```python
from build123d import *

# Parameters (mm, degrees)
SKETCH1_W           = 240
SKETCH1_H           = 45
SKETCH1_R           = 1.5
SKETCH1_W_2         = 5
SKETCH1_H_2         = 10
BOSS_EXTRUDE1_DEPTH = 5
CUT_EXTRUDE1_DEPTH  = 5
FILLET1_R           = 2
CONG_1_R            = 5


with BuildPart() as part:
    # Sketch1 → Boss-Extrude1 (new body)
    with BuildSketch(Plane.XY):
        with Locations((34.186746988, 0)):
            Rectangle(SKETCH1_W, SKETCH1_H)
        with Locations((-78.313253012, 0)):
            Circle(SKETCH1_R, mode=Mode.SUBTRACT)
        with Locations(Location((146.686746988, 0, 0), (0, 0, 180))):
            Circle(SKETCH1_R, mode=Mode.SUBTRACT)
        with Locations((-78.313253012, -15)):
            Rectangle(SKETCH1_W_2, SKETCH1_H_2, mode=Mode.SUBTRACT)
        with Locations((-78.313253012, 15)):
            Rectangle(SKETCH1_W_2, SKETCH1_H_2, mode=Mode.SUBTRACT)
        with Locations((146.686746988, -15)):
            Rectangle(SKETCH1_W_2, SKETCH1_H_2, mode=Mode.SUBTRACT)
        with Locations((146.686746988, 15)):
            Rectangle(SKETCH1_W_2, SKETCH1_H_2, mode=Mode.SUBTRACT)
    extrude(amount=BOSS_EXTRUDE1_DEPTH)

    # Sketch2 → Cut-Extrude1 (cut)
    with BuildSketch(Plane.XY.offset(5)):
        with BuildLine():
            Line((-68.813253012, 22.5), (-62.813253012, 22.5))
            Line((-62.813253012, 22.5), (-64.063253012, 10))
            ThreePointArc((-64.063253012, 10), (-65.813253012, 8.25), (-67.563253012, 10))
            Line((-67.563253012, 10), (-68.813253012, 22.5))
        make_face()
        with BuildLine():
            Line((-43.813253012, 22.5), (-37.813253012, 22.5))
            Line((-37.813253012, 22.5), (-39.063253012, 10))
            ThreePointArc((-39.063253012, 10), (-40.813253012, 8.25), (-42.563253012, 10))
            Line((-42.563253012, 10), (-43.813253012, 22.5))
        make_face()
        with BuildLine():
            Line((-18.813253012, 22.5), (-12.813253012, 22.5))
            Line((-12.813253012, 22.5), (-14.063253012, 10))
            ThreePointArc((-14.063253012, 10), (-15.813253012, 8.25), (-17.563253012, 10))
            Line((-17.563253012, 10), (-18.813253012, 22.5))
        make_face()
        with BuildLine():
            Line((6.186746988, 22.5), (12.186746988, 22.5))
            Line((12.186746988, 22.5), (10.936746988, 10))
            ThreePointArc((10.936746988, 10), (9.186746988, 8.25), (7.436746988, 10))
            Line((7.436746988, 10), (6.186746988, 22.5))
        make_face()
        with BuildLine():
            Line((31.186746988, 22.5), (37.186746988, 22.5))
            Line((37.186746988, 22.5), (35.936746988, 10))
            ThreePointArc((35.936746988, 10), (34.186746988, 8.25), (32.436746988, 10))
            Line((32.436746988, 10), (31.186746988, 22.5))
        make_face()
        with BuildLine():
            Line((56.186746988, 22.5), (62.186746988, 22.5))
            Line((62.186746988, 22.5), (60.936746988, 10))
            ThreePointArc((60.936746988, 10), (59.186746988, 8.25), (57.436746988, 10))
            Line((57.436746988, 10), (56.186746988, 22.5))
        make_face()
        with BuildLine():
            Line((81.186746988, 22.5), (87.186746988, 22.5))
            Line((87.186746988, 22.5), (85.936746988, 10))
            ThreePointArc((85.936746988, 10), (84.186746988, 8.25), (82.436746988, 10))
            Line((82.436746988, 10), (81.186746988, 22.5))
        make_face()
        with BuildLine():
            Line((106.186746988, 22.5), (112.186746988, 22.5))
            Line((112.186746988, 22.5), (110.936746988, 10))
            ThreePointArc((110.936746988, 10), (109.186746988, 8.25), (107.436746988, 10))
            Line((107.436746988, 10), (106.186746988, 22.5))
        make_face()
        with BuildLine():
            Line((131.186746988, 22.5), (137.186746988, 22.5))
            Line((137.186746988, 22.5), (135.936746988, 10))
            ThreePointArc((135.936746988, 10), (134.186746988, 8.25), (132.436746988, 10))
            Line((132.436746988, 10), (131.186746988, 22.5))
        make_face()
        with BuildLine():
            Line((137.186746988, -22.5), (135.936746988, -10))
            ThreePointArc((135.936746988, -10), (134.186746988, -8.25), (132.436746988, -10))
            Line((132.436746988, -10), (131.186746988, -22.5))
            Line((131.186746988, -22.5), (137.186746988, -22.5))
        make_face()
        with BuildLine():
            Line((112.186746988, -22.5), (110.936746988, -10))
            ThreePointArc((110.936746988, -10), (109.186746988, -8.25), (107.436746988, -10))
            Line((107.436746988, -10), (106.186746988, -22.5))
            Line((106.186746988, -22.5), (112.186746988, -22.5))
        make_face()
        with BuildLine():
            Line((87.186746988, -22.5), (85.936746988, -10))
            ThreePointArc((85.936746988, -10), (84.186746988, -8.25), (82.436746988, -10))
            Line((82.436746988, -10), (81.186746988, -22.5))
            Line((81.186746988, -22.5), (87.186746988, -22.5))
        make_face()
        with BuildLine():
            Line((62.186746988, -22.5), (60.936746988, -10))
            ThreePointArc((60.936746988, -10), (59.186746988, -8.25), (57.436746988, -10))
            Line((57.436746988, -10), (56.186746988, -22.5))
            Line((56.186746988, -22.5), (62.186746988, -22.5))
        make_face()
        with BuildLine():
            Line((37.186746988, -22.5), (35.936746988, -10))
            ThreePointArc((35.936746988, -10), (34.186746988, -8.25), (32.436746988, -10))
            Line((32.436746988, -10), (31.186746988, -22.5))
            Line((31.186746988, -22.5), (37.186746988, -22.5))
        make_face()
        with BuildLine():
            Line((12.186746988, -22.5), (10.936746988, -10))
            ThreePointArc((10.936746988, -10), (9.186746988, -8.25), (7.436746988, -10))
            Line((7.436746988, -10), (6.186746988, -22.5))
            Line((6.186746988, -22.5), (12.186746988, -22.5))
        make_face()
        with BuildLine():
            Line((-12.813253012, -22.5), (-14.063253012, -10))
            ThreePointArc((-14.063253012, -10), (-15.813253012, -8.25), (-17.563253012, -10))
            Line((-17.563253012, -10), (-18.813253012, -22.5))
            Line((-18.813253012, -22.5), (-12.813253012, -22.5))
        make_face()
        with BuildLine():
            Line((-37.813253012, -22.5), (-39.063253012, -10))
            ThreePointArc((-39.063253012, -10), (-40.813253012, -8.25), (-42.563253012, -10))
            Line((-42.563253012, -10), (-43.813253012, -22.5))
            Line((-43.813253012, -22.5), (-37.813253012, -22.5))
        make_face()
        with BuildLine():
            Line((-62.813253012, -22.5), (-64.063253012, -10))
            ThreePointArc((-64.063253012, -10), (-65.813253012, -8.25), (-67.563253012, -10))
            Line((-67.563253012, -10), (-68.813253012, -22.5))
            Line((-68.813253012, -22.5), (-62.813253012, -22.5))
        make_face()
    extrude(amount=-CUT_EXTRUDE1_DEPTH, mode=Mode.SUBTRACT)

    # Fillet1
    fillet1_edges = [part.edges().sort_by_distance(p)[0] for p in [
        (-62.813253012, -22.5, 2.5),
        (-68.813253012, -22.5, 2.5),
        (-37.813253012, -22.5, 2.5),
        (-43.813253012, -22.5, 2.5),
        (-12.813253012, -22.5, 2.5),
        (-18.813253012, -22.5, 2.5),
        (12.186746988, -22.5, 2.5),
        (6.186746988, -22.5, 2.5),
        (37.186746988, -22.5, 2.5),
        (31.186746988, -22.5, 2.5),
        (62.186746988, -22.5, 2.5),
        (56.186746988, -22.5, 2.5),
        (87.186746988, -22.5, 2.5),
        (81.186746988, -22.5, 2.5),
        (112.186746988, -22.5, 2.5),
        (106.186746988, -22.5, 2.5),
        (137.186746988, -22.5, 2.5),
        (131.186746988, -22.5, 2.5),
        (131.186746988, 22.5, 2.5),
        (137.186746988, 22.5, 2.5),
        (106.186746988, 22.5, 2.5),
        (112.186746988, 22.5, 2.5),
        (81.186746988, 22.5, 2.5),
        (87.186746988, 22.5, 2.5),
        (56.186746988, 22.5, 2.5),
        (62.186746988, 22.5, 2.5),
        (31.186746988, 22.5, 2.5),
        (37.186746988, 22.5, 2.5),
        (6.186746988, 22.5, 2.5),
        (12.186746988, 22.5, 2.5),
        (-18.813253012, 22.5, 2.5),
        (-12.813253012, 22.5, 2.5),
        (-43.813253012, 22.5, 2.5),
        (-37.813253012, 22.5, 2.5),
        (-68.813253012, 22.5, 2.5),
        (-62.813253012, 22.5, 2.5),
    ]]
    fillet(fillet1_edges, radius=FILLET1_R)

    # Congé1
    cong_1_edges = [part.edges().sort_by_distance(p)[0] for p in [
        (-85.813253012, 22.5, 2.5),
        (154.186746988, 22.5, 2.5),
        (154.186746988, -22.5, 2.5),
        (-85.813253012, -22.5, 2.5),
    ]]
    fillet(cong_1_edges, radius=CONG_1_R)


solid = part.part
```
Geometry check sheet. Reference: the model listing, model coordinates, mm. A direction names the side the tool comes from. Give positions to 0.01 mm unless a question says otherwise; leave off trailing zeros. Use a Markdown table: item, result.
Q1. Go/stop test with a flat-tipped pin: P1, Ø10, axis at x = -55, y = 14.5, coming from the -Z side. Record where the tip stops, or that it passes through.
Computed:
| item | result |
|---|---|
| P1 | stops at z = 0 |
Q2. Draft check along X on faces 6 (the face through (22, -22.5, 2)), 7 (the face through (-80.813, -15, 2)). Enter one of: pulls with the +X half, pulls with the -X half, needs draft (parallel to the pull), parting line crosses it, or undercut.
Computed:
| item | result |
|---|---|
| face 6 | needs draft |
| face 7 | undercut |
Q3. Section check A-A, the plane z = 3.9. Give the number of separate pieces and of enclosed holes in the cut face, then the cut area to 3 significant figures.
Computed:
| item | result |
|---|---|
| separate pieces | 1 |
| enclosed holes | 6 |
| area | 9,380 mm² |
Q4. Thickness scan on L1, parallel to Y at x = 110.5, z = 1.95. Record the ranges inside material, lowest first. Write a range as [from, to].
Computed:
| item | result |
|---|---|
| L1 | y = [-8.84, 8.84] |
Q5. Set-up check for faces 1 (the face through (136.48, 15.42, 2.54)), 2 (the face through (36.48, -15.42, 2.54)), 3 (the face through (33, 0, 0)), 4 (the face through (-76, -22.5, 2)), 5 (the face through (149.187, 15, 2)): record each of +Z, -Z, +X, -X, +Y, -Y from which the full face is reachable in a straight line by a thin tool's end or side.
Computed:
| item | result |
|---|---|
| face 1 | +Z, -Z, +Y |
| face 2 | +Z, -Z, -Y |
| face 3 | -Z, +X, -X, +Y, -Y |
| face 4 | +Z, -Z, +X, -X, -Y |
| face 5 | +Z, -Z |
